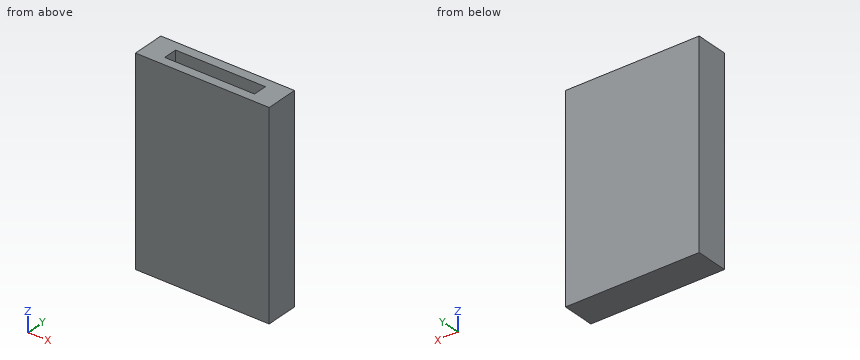
Autodesk Inventor part; units mm, degrees
ref_plane "YZ Plane" through (0, 0, 0) normal (1, 0, 0) x (0, 1, 0)
ref_plane "XZ Plane" through (0, 0, 0) normal (0, 1, 0) x (-1, 0, 0)
ref_plane "XY Plane" through (0, 0, 0) normal (0, 0, 1) x (1, 0, 0)
sketch "Sketch1" plane through (0, 0, 0) normal (0, 0, 1) x (1, 0, 0)
  line L0 (-5.4331, 6.9327) -> (4.5669, 6.9327)
  line L1 (4.5669, 6.9327) -> (4.5669, 4.4986)
  line L2 (4.5669, 4.4986) -> (-5.4331, 4.4986)
  line L3 (-5.4331, 4.4986) -> (-5.4331, 6.9327)
  point P0 (0, 0)
  dimension "d0" = 10
extrude "Extrusion1" add sketch "Sketch1" along normal blind 15
sketch "Sketch2" plane through (0, 0, 15) normal (0, 0, 1) x (1, 0, 0)
  line L0 (-3.7689, 6.2173) -> (2.9461, 6.2173)
  line L1 (2.9461, 6.2173) -> (2.9461, 5.1689)
  line L2 (2.9461, 5.1689) -> (-3.7689, 5.1689)
  line L3 (-3.7689, 5.1689) -> (-3.7689, 6.2173)
  point P0 (0, 0)
extrude "Extrusion2" cut sketch "Sketch2" against normal blind 1.5
properties part number "cutter grp 17-2"
The listing builds one solid part. Answer for the finished solid, in the listing's coordinates (mm). Coordinates: 2 decimals unless noted, no trailing zeros. Loops run counter-clockwise (first coordinate to the right, second up) from the corner with the lowest first, then second, coordinate; pieces in that order, holes last. Notation, with made-up numbers: M 17.5,33.5 L 35.5,33.5 A15 ccw 35.5,48.5 Z; hole C 12.25,70.5 d4. An arc over 180 degrees is marked long. Answer as CSV lines item,"result". Start each with the question number.
(1) The part is cut by section A-A (z = 14). Give the vertices of the cut face in (x, y), and give its area (3 significant figures).
(2) Find the intervals of material crossed by L1, parallel to Z at x = -0.75, y = 5.9, in increasing order. Write a range as [from, to].
(3) Given pin 1 (0.5 mm diameter, centred on x = 0, y = 5.5, fed in from +Z), flat-ended and moving along its own axis, determine where the tip first touches the part or whether it passes through.
(4) The part is cut by section B-B (x = -1). Give the vertices of the cut face in (y, z).
Determined:
1,outline,"M -5.43,4.5 L 4.57,4.5 L 4.57,6.93 L -5.43,6.93 Z; hole M -3.77,5.17 L 2.95,5.17 L 2.95,6.22 L -3.77,6.22 Z"
1,area,"17.3 mm2"
2,L1,"[0, 13.5]"
3,pin 1,"z = 13.5"
4,outline,"M 4.5,0 L 6.93,0 L 6.93,15 L 6.22,15 L 6.22,13.5 L 5.17,13.5 L 5.17,15 L 4.5,15 Z"
